```python
from build123d import *

# Parameters (mm, degrees)
SKETCH1_W           = 21.59
SKETCH1_H           = 5.334
BOSS_EXTRUDE1_DEPTH = 5.334
SKETCH2_R           = 18.1
CUT_EXTRUDE1_DEPTH  = 5.334


with BuildPart() as part:
    # Sketch1 → Boss-Extrude1 (new body)
    with BuildSketch(Plane.XY):
        Polygon((-36.2, 24.449992223), (-23.5, 24.449992223), (-23.5, 42.483992223), (23.49, 42.483992223), (23.49, 24.449992223), (36.2, 24.449992223), (36.2, -7.777e-06), (18.1, -26.619054692), (-18.1, -26.619054692), (-36.2, 2.462571049), align=None)
        with Locations((-0.005, 32.451)):
            Rectangle(SKETCH1_W, SKETCH1_H, mode=Mode.SUBTRACT)
    extrude(amount=BOSS_EXTRUDE1_DEPTH)

    # Sketch2 → Cut-Extrude1 (cut)
    with BuildSketch(Plane.XY.offset(5.334)):
        Circle(SKETCH2_R)
    extrude(amount=-CUT_EXTRUDE1_DEPTH, mode=Mode.SUBTRACT)


solid = part.part
```
Here's how the part is built. I have some questions about the finished solid (model axes, mm). A direction names the side the tool comes from. Give positions to 0.01 mm unless a question says otherwise; leave off trailing zeros. Write each loop counter-clockwise with the first axis right and the second up, starting at its lowest first coordinate (ties: lowest second). Pieces come first, ordered by that corner, then holes. Notation, with made-up numbers: M 68,23.5 L 118,23.5 A18 ccw 118,40.5 Z; hole C -3.75,55 d6. An arc over 180 degrees is marked long. Put each result on its own line as item: value. Start each with the question number.
Item 1: If we section it at A-A, the plane x = 0: Write out the boundary of the cut face in (y, z), then the cut area to 3 significant figures.
Item 2: I need wall thicknesses on L1, parallel to Y at x = 0, z = 3.65; L2, parallel to X at y = 33.5, z = 1.45; L3, parallel to Y at x = 10, z = 0.7. Which ranges of each line are inside material? Lowest first, please. Write a range as from..to.
Item 3: If we section it at D-D, the plane y = 37: Write out the boundary of the cut face in (x, z), then the cut area to 3 significant figures.
Item 4: If we section it at B-B, the plane z = 2.25: Write out the boundary of the cut face in (x, y).
Item 5: Thinking about a two-plate mould opening in Y: for faces 4 (the flat face through (0, 35.118, 3)), 5 (the flat face through (-30, 24.45, 3)), 6 (the flat face through (-27.023, -12.282, 2.63)), which applies, +Y half, -Y half, draft (parallel to the pull), parting line (faces both ways), or undercut?
Item 6: If we section it at C-C, the plane y = 11.5: Write out the boundary of the cut face in (x, z), then the cut area to 3 significant figures.
Item 7: Will these pins go through, and if not, where does the flat tip stop? pin 1 (1.6 mm diameter, centred on x = 29, z = 4, fed in from +Y); pin 2 (2.5 mm diameter, centred on y = 33, z = 2.5, fed in from +X); pin 3 (2.5 mm diameter, centred on y = 31.5, z = 2, fed in from -X).
Item 8: On a 3-axis mill with a long thin cutter (end or side, diameter ignored), from which of +Z, -Z, +X, -X, +Y, -Y can I reach the whole of each face in a straight line? I mean faces 1 (the flat face through (-23.5, 33, 3)), 2 (the flat face through (0, 29.784, 3)), 3 (the flat face through (30, 24.45, 3)). Say none if no direction works.
Values:
1. outline: M -26.62,0 L -18.1,0 L -18.1,5.33 L -26.62,5.33 Z; M 18.1,0 L 29.78,0 L 29.78,5.33 L 18.1,5.33 Z; M 35.12,0 L 42.48,0 L 42.48,5.33 L 35.12,5.33 Z
1. area: 147 mm²
2. L1: -26.62..-18.1, 18.1..29.78, 35.12..42.48
2. L2: -23.5..-10.8, 10.79..23.49
2. L3: -26.62..-15.09, 15.09..29.78, 35.12..42.48
3. outline: M -23.5,0 L 23.49,0 L 23.49,5.33 L -23.5,5.33 Z
3. area: 251 mm²
4. outline: M -36.2,2.46 L -18.1,-26.62 L 18.1,-26.62 L 36.2,0 L 36.2,24.45 L 23.49,24.45 L 23.49,42.48 L -23.5,42.48 L -23.5,24.45 L -36.2,24.45 Z; hole C 0,0 d36.2; hole M -10.8,29.78 L 10.79,29.78 L 10.79,35.12 L -10.8,35.12 Z
5. face 4: undercut
5. face 5: +Y half
5. face 6: -Y half
6. outline: M -36.2,0 L -13.98,0 L -13.98,5.33 L -36.2,5.33 Z; M 13.98,0 L 36.2,0 L 36.2,5.33 L 13.98,5.33 Z
6. area: 237 mm²
7. pin 1: y = 24.45
7. pin 2: x = 23.49
7. pin 3: x = -23.5
8. face 1: +Z, -Z, -X, +Y
8. face 2: +Z, -Z
8. face 3: +Z, -Z, +X, +Y
